from build123d import *

# Parameters (mm, degrees)
SKETCH1_R           = 1.66
SKETCH1_R_2         = 1.15
SKETCH1_R_3         = 1.4
BOSS_EXTRUDE1_DEPTH = 1.25
FILLET1_R           = 5


with BuildPart() as part:
    # Sketch1 → Boss-Extrude1 (new body)
    with BuildSketch(Plane(origin=(0, 0, 0), x_dir=(1, 0, 0), z_dir=(0, 1, 0))):
        Polygon((-14.713467049, 74.209885387), (-14.713467049, -22.790114613), (12.786532951, -22.790114613), (12.786532951, -7.790114613), (37.786532951, -7.790114613), (37.786532951, 74.209885387), align=None)
        with Locations(Location((-9.713467049, 65.709885387, 0), (0, 0, 270))):  # turned: the seam where the file's is
            Circle(SKETCH1_R, mode=Mode.SUBTRACT)
        with Locations(Location((1.786532951, 65.709885387, 0), (0, 0, 270))):  # turned: the seam where the file's is
            Circle(SKETCH1_R_2, mode=Mode.SUBTRACT)
        with Locations(Location((20.786532951, 65.709885387, 0), (0, 0, 270))):  # turned: the seam where the file's is
            Circle(SKETCH1_R_2, mode=Mode.SUBTRACT)
        with Locations(Location((1.786532951, 53.209885387, 0), (0, 0, 270))):  # turned: the seam where the file's is
            Circle(SKETCH1_R, mode=Mode.SUBTRACT)
        with Locations(Location((1.786532951, 25.709885387, 0), (0, 0, 270))):  # turned: the seam where the file's is
            Circle(SKETCH1_R, mode=Mode.SUBTRACT)
        with Locations(Location((20.786532951, 53.209885387, 0), (0, 0, 270))):  # turned: the seam where the file's is
            Circle(SKETCH1_R, mode=Mode.SUBTRACT)
        with Locations(Location((20.786532951, 25.709885387, 0), (0, 0, 270))):  # turned: the seam where the file's is
            Circle(SKETCH1_R, mode=Mode.SUBTRACT)
        with Locations(Location((1.786532951, -3.290114613, 0), (0, 0, 270))):  # turned: the seam where the file's is
            Circle(SKETCH1_R_2, mode=Mode.SUBTRACT)
        with Locations(Location((20.786532951, -3.290114613, 0), (0, 0, 270))):  # turned: the seam where the file's is
            Circle(SKETCH1_R_2, mode=Mode.SUBTRACT)
        with Locations(Location((-9.713467049, -3.290114613, 0), (0, 0, 270))):  # turned: the seam where the file's is
            Circle(SKETCH1_R, mode=Mode.SUBTRACT)
        with Locations(Location((7.786532951, -19.040114613, 0), (0, 0, 270))):  # turned: the seam where the file's is
            Circle(SKETCH1_R_3, mode=Mode.SUBTRACT)
    extrude(amount=BOSS_EXTRUDE1_DEPTH)

    # Fillet1
    fillet1_edges = [part.edges().sort_by_distance(p)[0] for p in [
        (-14.713467049, 0.625, -74.209885387),
    ]]
    fillet(fillet1_edges, radius=FILLET1_R)


solid = part.part
The listing builds one solid part. Answer for the finished solid, in the listing's coordinates (mm). Round coordinates to 2 decimals unless told otherwise and drop trailing zeros. Order: outer loops, then holes, each group sorted by start corner. A loop starts at its lowest first (then second) coordinate and runs counter-clockwise, first axis right, second up. Notation, with made-up numbers: M 18,-23.75 L 74,-23.75 A29 cw 74,15.25 Z; hole C -32,19 d1. An arc over 180 degrees is marked long. Answer in a Markdown table with one row per item. Add a question column.
1) Consider line 1 along X through (y, z) = (1.2, -53); line 2 along Z through (x, y) = (21, 0.1); line 3 along Z through (x, y) = (20.5, 1.05). Determine where each line is inside the solid, lowest interval first. Write a range as from..to.
2) The part is cut by section A-A on y = 0.65. Count the separate pieces of the cut face and the enclosed holes in it, plus the area to 3 significant figures.
3) Flat-ended cylindrical pins translate along their axes: pin 1 Ø1.4 at (x, z) = (20.79, 3.29) entering from +Y; pin 2 Ø0.6 at (x, y) = (22.5, 0.5) entering from +Z. Find the tip coordinate at first contact, or state that the pin passes through.
4) The part is cut by section B-B on x = 16. Determine the outline of the cut face in (y, z).
5) Determine the mould class of faces 1 (the face through (-13.288, 0.634, -72.706)), 2 (the face through (19.766, 0.616, 3.821)), 3 (the face through (11, 0, -26)), 4 (the face through (0.78, 0.62, -54.53)) for opening direction X: pulls with the +X half, pulls with the -X half, needs draft (parallel to the pull), parting line crosses it, or undercut.
Findings below:
| question | item | result |
|---|---|---|
| 1 | line 1 | x = -14.71..0.14, 3.43..19.14, 22.43..37.79 |
| 1 | line 2 | z = -74.21..-66.84, -64.58..-54.86, -51.56..-27.36, -24.06..2.16, 4.42..7.79 |
| 1 | line 3 | z = -74.21..-66.82, -64.6..-54.84, -51.57..-27.34, -24.07..2.18, 4.4..7.79 |
| 2 | separate pieces | 1 |
| 2 | enclosed holes | 11 |
| 2 | area | 4,640 mm² |
| 3 | pin 1 | passes through |
| 3 | pin 2 | stops at z = 7.79 |
| 4 | outline | M 0,-74.21 L 1.25,-74.21 L 1.25,7.79 L 0,7.79 Z |
| 5 | face 1 | pulls with the -X half |
| 5 | face 2 | undercut |
| 5 | face 3 | needs draft |
| 5 | face 4 | undercut |
